CAD build for the part. Positions are in the model's coordinates, mm. Face numbers are marked on the shaded views. A direction names the side the tool comes from. Round coordinates to 2 decimals unless told otherwise and drop trailing zeros. Write each loop counter-clockwise with the first axis right and the second up, starting at its lowest first coordinate (ties: lowest second). Pieces come first, ordered by that corner, then holes. Notation, with made-up numbers: (46, -18.5) - (88, -18.5) arc R10 ccw to (88, -9.5) - close; hole circle Ø6 at (44, 1.25). An arc over 180 degrees is marked (long way). Answer in a Markdown table with one row per item.
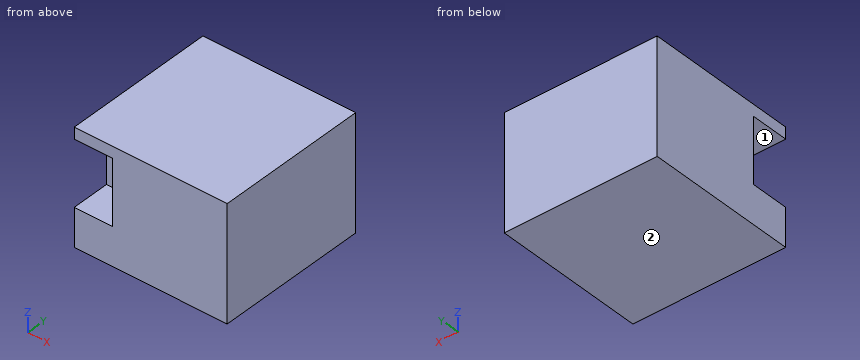
```python
from build123d import *

# Parameters (mm, degrees)
BOSS_EXTRUDE1_DEPTH      = 15
BOSS_EXTRUDE1_DEPTH_BACK = 15
SKETCH1_W                = 40
SKETCH1_H                = 40
CUT_EXTRUDE1_DEPTH       = 12
CUT_EXTRUDE1_DEPTH_BACK  = 5
SKETCH2_W                = 10
SKETCH2_H                = 10


with BuildPart() as part:
    # Sketch1 → Boss-Extrude1 (new, two sides: drawn at the far end of the back side and taken through both)
    with BuildSketch(Plane.XY.offset(-BOSS_EXTRUDE1_DEPTH_BACK)):
        with Locations((20, 20)):
            Rectangle(SKETCH1_W, SKETCH1_H)
    extrude(amount=BOSS_EXTRUDE1_DEPTH + BOSS_EXTRUDE1_DEPTH_BACK)

    # Sketch2 → Cut-Extrude1 (cut, two sides: drawn at the far end of the back side and taken through both)
    with BuildSketch(Plane.XY.offset(-CUT_EXTRUDE1_DEPTH_BACK)):
        with Locations((5, 5)):
            Rectangle(SKETCH2_W, SKETCH2_H)
    extrude(amount=CUT_EXTRUDE1_DEPTH + CUT_EXTRUDE1_DEPTH_BACK, mode=Mode.SUBTRACT)


solid = part.part
```
Q1. Flat gauge pin, fed straight in: pin 1 (3 mm diameter, centred on x = 4, z = 1, fed in from -Y). Where does the tip first touch, or does it go through?
Computed:
| item | result |
|---|---|
| pin 1 | stops at y = 10 |
Q2. Saw through at A-A on x = 5.5. List the corners of the cut face in (y, z), then the cut area to 3 significant figures.
Computed:
| item | result |
|---|---|
| outline | (0, -15) - (40, -15) - (40, 15) - (0, 15) - (0, 12) - (10, 12) - (10, -5) - (0, -5) - close |
| area | 1,030 mm2 |
Q3. 3-axis set-ups, long thin cutter, end or side, ignore diameter. For the marked faces 1 and 2: which of +Z, -Z, +X, -X, +Y, -Y reach the whole face in a straight line?
Computed:
| item | result |
|---|---|
| face 1 | -X, -Y |
| face 2 | -Z, +X, -X, +Y, -Y |
Q4. Saw through at C-C on z = 3.25. List the corners of the cut face in (x, y), then the cut area to 3 significant figures.
Computed:
| item | result |
|---|---|
| outline | (0, 10) - (10, 10) - (10, 0) - (40, 0) - (40, 40) - (0, 40) - close |
| area | 1,500 mm2 |
Q5. Drill centre line: line 1 (Y direction, x = 8, z = 2.25). Where is it in solid material? Low to high.
Computed:
| item | result |
|---|---|
| line 1 | y = 10 to 40 |
